```python
from build123d import *

# Parameters (mm, degrees)
SKETCH2_W                = 10
SKETCH2_H                = 10
BOSS_EXTRUDE1_DEPTH      = 2
M2_CLEARANCE_HOLE1_D     = 2.4
M2_CLEARANCE_HOLE1_DEPTH = 2
M2_CLEARANCE_HOLE1_TIP   = 0.721032743
SKETCH5_W                = 10
SKETCH5_H                = 2
BOSS_EXTRUDE2_DEPTH      = 10
SWEEP1_START             = -5
SWEEP1_DEPTH             = 10
M2_CLEARANCE_HOLE2_D     = 2.4


# Read off the part's stored shape, not the designer's step: Sweep1
with BuildPart() as part:
    # Sketch2 → Boss-Extrude1 (new body)
    with BuildSketch(Plane(origin=(0, 0, 0), x_dir=(1, 0, 0), z_dir=(0, 1, 0))):
        Rectangle(SKETCH2_W, SKETCH2_H)
    extrude(amount=BOSS_EXTRUDE1_DEPTH)

    # M2 Clearance Hole1
    with Locations(Plane(origin=(0, 0, 0), x_dir=(-1, 0, 0), z_dir=(0, -1, 0))):
        with Locations((0, -1)):
            Hole(M2_CLEARANCE_HOLE1_D / 2, depth=M2_CLEARANCE_HOLE1_DEPTH)
            with Locations((0, 0, -(M2_CLEARANCE_HOLE1_DEPTH + M2_CLEARANCE_HOLE1_TIP / 2))):  # 118° drill point
                Cone(0, M2_CLEARANCE_HOLE1_D / 2, M2_CLEARANCE_HOLE1_TIP, mode=Mode.SUBTRACT)

    # Sketch5 → Boss-Extrude2 (add)
    with BuildSketch(Plane(origin=(0, 2, 0), x_dir=(1, 0, 0), z_dir=(0, 1, 0))):
        with Locations((0, 4)):
            Rectangle(SKETCH5_W, SKETCH5_H)
    extrude(amount=BOSS_EXTRUDE2_DEPTH)

    # Sweep1 outline → Sweep1 (add)
    with BuildSketch(Plane.YZ.offset(SWEEP1_START)):
        with BuildLine():
            add(Edge.make_bspline(
                [(12, -3), (22.081437319, -3.280824846), (30.428491616, -1.29359039), (43.829554593, 7.091969611), (48.931984519, 13.47592334), (52.477312717, 22.194576498)],
                knots=[0, 0, 0, 0, 0.5, 0.5, 0.99708935, 0.99708935, 0.99708935, 0.99708935], degree=3))
            Line((12, -3), (12, -5))
            add(Edge.make_bspline(
                [(12, -5), (22.363265836, -5.280469752), (31.151391085, -3.215010639), (41.80972213, 3.477460348), (44.938271104, 6.304066685), (48.978333418, 11.413324262), (50.216569106, 13.261147564), (52.476984989, 17.242675991), (53.506405959, 19.395799121), (54.435317643, 21.703901173), (54.455920091, 21.755052947), (54.476559414, 21.806291518)],
                knots=[0, 0, 0, 0, 0.5, 0.5, 0.75, 0.75, 0.875, 0.875, 1, 1, 1.002873769, 1.002873769, 1.002873769, 1.002873769], degree=3))
            Line((54.476559414, 21.806291518), (54.476559414, 31.827443689))
            Line((54.476559414, 31.827443689), (52.477312712, 31.772556311))
            Line((52.477312712, 31.772556311), (52.477312717, 22.194576498))
        make_face()
    extrude(amount=SWEEP1_DEPTH)

    # M2 Clearance Hole2 (through all)
    with Locations(Plane(origin=(0, 52.477312712, 0), x_dir=(-1, 0, 0), z_dir=(0, -1, 0))):
        with Locations((0, -29.772556311)):
            Hole(M2_CLEARANCE_HOLE2_D / 2)


solid = part.part
```
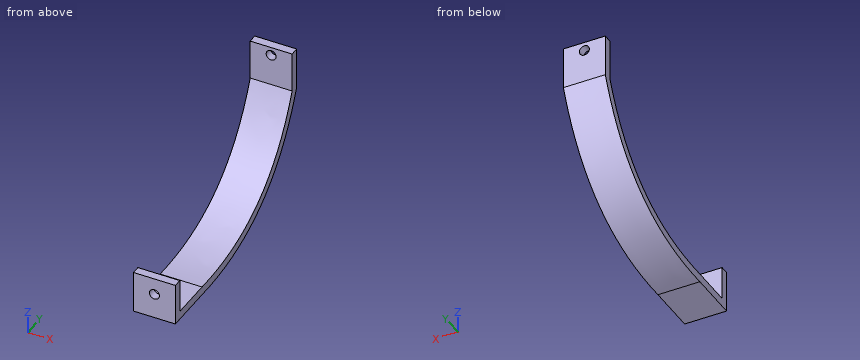
Here's how the part is built. I have some questions about the finished solid (model axes, mm). Give positions to 0.01 mm unless a question says otherwise; leave off trailing zeros. Loops run counter-clockwise (first coordinate to the right, second up) from the corner with the lowest first, then second, coordinate; pieces in that order, holes last. Notation, with made-up numbers: M 12.5,-19.75 L 21.5,-19.75 A24 cw 21.5,11.25 Z; hole C 28,-11.5 d11. An arc over 180 degrees is marked long. Return JSON: item names as keys, results as strings.
Item 1: I'm going to push flat-ended pins straight in: pin 1 Ø3 at (x, y) = (0.5, 5) entering from +Z; pin 2 Ø3 at (x, y) = (2.5, 47.5) entering from +Z; pin 3 Ø1 at (x, y) = (-1, 36.5) entering from -Z. Where does each tip first touch, or does it pass through?
A:
{"pin 1": "stops at z = -3", "pin 2": "stops at z = 15.2", "pin 3": "stops at z = -0.06"}
Item 2: Imagine slicing it at A-A on x = 0. State how many separate pieces and enclosed holes the cut face has, then the cut area to 3 significant figures.
A:
{"separate pieces": "3", "enclosed holes": "0", "area": "155 mm^2"}
Item 3: Please list where these lines run through material, in increasing order: line 1 (Z direction, x = 0, y = 0.55); line 2 (Y direction, x = -2, z = 2); line 3 (Z direction, x = 0, y = 54).
A:
{"line 1": "z = -5 to -0.2, 2.2 to 5", "line 2": "y = 0 to 2, 35.6 to 39.41", "line 3": "z = 20.65 to 28.57, 30.97 to 31.81"}
Item 4: Imagine slicing it at B-B on z = 27.5. List the corners of the cut face in (x, y) for me.
A:
{"outline": "M -5,52.48 L 5,52.48 L 5,54.48 L -5,54.48 Z"}
